```python
from build123d import *

# Parameters (mm, degrees)
PAD_DEPTH    = 36
SKETCH001_R  = 1.6
POCKET_DEPTH = 10


with BuildPart() as part:
    # Sketch → Pad (new body)
    with BuildSketch(Plane.XY):
        with BuildLine():
            ThreePointArc((2.201846, -3.339442), (0.011769, 3.999983), (-2.22146, -3.326427))
            ThreePointArc((-2.22146, -3.326427), (-1.387999, -3.751461), (-0.478604, -3.971264))
            Line((-0.478604, -3.971264), (-0.478604, -11.086475))
            Line((-0.478604, -11.086475), (-1.32632, -11.086475))
            Line((-1.32632, -5.816765), (-1.32632, -11.086475))
            ThreePointArc((-2.084926, 5.589898), (-5.95291, -0.395901), (-1.32632, -5.816765))
            Line((-18, 5.589898), (-2.084926, 5.589898))
            Line((-18, 5.589898), (-18, 9.589898))
            Line((-18, 9.589898), (18, 9.589898))
            Line((18, 9.589898), (18, 5.589898))
            Line((2.084926, 5.589898), (18, 5.589898))
            ThreePointArc((1.451052, -5.78691), (5.956822, -0.331892), (2.084926, 5.589898))
            Line((1.451052, -5.78691), (1.451052, -11.069447))
            Line((0.603336, -11.069447), (1.451052, -11.069447))
            Line((0.603336, -3.954236), (0.603336, -11.069447))
            ThreePointArc((0.603336, -3.954236), (1.435881, -3.733396), (2.201846, -3.339442))
        make_face()
    extrude(amount=PAD_DEPTH)

    # Sketch001 → Pocket (cut)
    with BuildSketch(Plane(origin=(0, 9.589898, 0), x_dir=(-1, 0, 0), z_dir=(0, 1, 0))):
        with Locations((-14.335366, 32.630134)):
            Circle(SKETCH001_R)
        with Locations((14.464634, 32.630134)):
            Circle(SKETCH001_R)
        with Locations((14.464634, 3.830134)):
            Circle(SKETCH001_R)
        with Locations((-14.335366, 3.830134)):
            Circle(SKETCH001_R)
    extrude(amount=-POCKET_DEPTH, mode=Mode.SUBTRACT)


solid = part.part
```
For this review, take the finished solid that the model builds, in its own axes (mm). A direction names the side the tool comes from. Round coordinates to 2 decimals unless told otherwise and drop trailing zeros. Order: outer loops, then holes, each group sorted by start corner. A loop starts at its lowest first (then second) coordinate and runs counter-clockwise, first axis right, second up. Notation, with made-up numbers: (-11.75, 54) -> (4.25, 54) arc R14 cw to (4.25, 69) -> close; hole circle Ø10 at (37.25, 54.5). An arc over 180 degrees is marked (long way). Use a Markdown table: item, result.
Item 1: Draft analysis for pull direction X (two halves, no side actions). For faces 4 (the flat face through (18, 8, 18)), 5 (the cylindrical face through (-12.866, 7.618, 3.9)), 6 (the cylindrical face through (15.515, 7.618, 4.911)), 7 (the flat face through (0, 5, 36)), state which applies: +X half, -X half, draft (parallel to the pull), parting line (faces both ways), or undercut.
Resolved:
| item | result |
|---|---|
| face 4 | +X half |
| face 5 | undercut |
| face 6 | undercut |
| face 7 | draft |
Item 2: Take a section at C-C (z = 15.5). State the section outline as (x, y) points.
Resolved:
| item | result |
|---|---|
| outline | (-18, 5.59) -> (-2.08, 5.59) arc R5.97 ccw to (-1.33, -5.82) -> (-1.33, -11.09) -> (-0.48, -11.09) -> (-0.48, -3.97) arc R4 cw to (-2.22, -3.33) arc R4 cw (long way) to (2.2, -3.34) arc R4 cw to (0.6, -3.95) -> (0.6, -11.07) -> (1.45, -11.07) -> (1.45, -5.79) arc R5.97 ccw to (2.08, 5.59) -> (18, 5.59) -> (18, 9.59) -> (-18, 9.59) -> close |
Item 3: Take a section at B-B (x = 15). State the section outline as (y, z) points.
Resolved:
| item | result |
|---|---|
| outline | (5.59, 0) -> (9.59, 0) -> (9.59, 2.37) -> (5.59, 2.37) -> close; (5.59, 5.29) -> (9.59, 5.29) -> (9.59, 31.17) -> (5.59, 31.17) -> close; (5.59, 34.09) -> (9.59, 34.09) -> (9.59, 36) -> (5.59, 36) -> close |
Item 4: Machinability: for faces 1 (the flat face through (1.451, -8, 18)), 2 (the flat face through (10, 5.59, 18)), 3 (the flat face through (-1.326, -8, 18)), which of the approach directions +Z, -Z, +X, -X, +Y, -Y give a long, thin tool a straight path to every point of the face, cutting with its end or side? Answer none if there is none.
Resolved:
| item | result |
|---|---|
| face 1 | +Z, -Z, +X, -Y |
| face 2 | +Z, -Z, +X |
| face 3 | +Z, -Z, -X, -Y |
Item 5: Take a section at D-D (y = -8.5). State the section outline as (x, z) points.
Resolved:
| item | result |
|---|---|
| outline | (-1.33, 0) -> (-0.48, 0) -> (-0.48, 36) -> (-1.33, 36) -> close; (0.6, 0) -> (1.45, 0) -> (1.45, 36) -> (0.6, 36) -> close |
Item 6: For pin 1 (0.7 mm diameter, centred on x = 1, z = 20, fed in from -Y); pin 2 (5 mm diameter, centred on y = 3, z = 5, fed in from +X); pin 3 (2.5 mm diameter, centred on y = -9.5, z = 24.5, fed in from +X), all flat-tipped, find the tip position at first contact; note any pin that passes through.
Resolved:
| item | result |
|---|---|
| pin 1 | stops at y = -11.07 |
| pin 2 | stops at x = 5.95 |
| pin 3 | stops at x = 1.45 |
Item 7: For line 1 along Z through (x, y) = (-14.5, 8.75); line 2 along Y through (x, z) = (0, 25.5); line 3 along X through (y, z) = (7.25, 3.5), list the stretches that pass through material, from the lowest coordinate up. Write a range as [from, to].
Resolved:
| item | result |
|---|---|
| line 1 | z = [0, 2.23], [5.43, 31.03], [34.23, 36] |
| line 2 | y = [4, 9.59] |
| line 3 | x = [-18, -16.03], [-12.9, 12.77], [15.9, 18] |
Item 8: Take a section at A-A (y = 0). State the section outline as (x, z) points.
Resolved:
| item | result |
|---|---|
| outline | (-5.97, 0) -> (-4, 0) -> (-4, 36) -> (-5.97, 36) -> close; (4, 0) -> (5.97, 0) -> (5.97, 36) -> (4, 36) -> close |
